Read the model definition and answer for the solid it produces. Units are mm, in the model's axes. Face numbers are marked on the shaded views. A direction names the side the tool comes from. Coordinates: 2 decimals unless noted, no trailing zeros. Order: outer loops, then holes, each group sorted by start corner. A loop starts at its lowest first (then second) coordinate and runs counter-clockwise, first axis right, second up. Notation, with made-up numbers: M 49.5,44.25 L 91.5,44.25 A12 cw 91.5,55.25 Z; hole C 18.5,4 d6. An arc over 180 degrees is marked long. Put each result on its own line as item: value.
from build123d import *

# Parameters (mm, degrees)
F0_W      = 76.2
F0_H      = 76.2
F1_DEPTH  = 25.4
F1_FACE_W = 76.2
F1_FACE_H = 76.2
F2_DEPTH  = 50.8
F3_R      = 25.4
F4_DEPTH  = 25.4
F5_R      = 25.4
F6_DEPTH  = 25.4
F7_W      = 38.1
F7_H      = 38.1
F8_DEPTH  = 101.6


with BuildPart() as f1:
    # F0 (on Front) → F1 (new body)
    with BuildSketch(Plane.XZ):
        with Locations((-36.805706, 34.59075)):
            Rectangle(F0_W, F0_H)
    extrude(amount=F1_DEPTH)

    # F1_face (on face) → F2 (join)
    with BuildSketch(Plane(origin=(-36.805706, -25.4, 34.59075), x_dir=(1, 0, 0), z_dir=(0, -1, 0))):
        Rectangle(F1_FACE_W, F1_FACE_H)
    extrude(amount=F2_DEPTH)

    # F3 (on face) → F4 (join)
    with BuildSketch(Plane.XZ.offset(76.2)):
        with Locations((-36.805706, 34.59075)):
            Circle(F3_R)
    extrude(amount=F4_DEPTH)

    # F5 (on face) → F6 (join)
    with BuildSketch(Plane.YZ.offset(1.294294)):
        with Locations((-38.1, 34.59075)):
            Circle(F5_R)
    extrude(amount=F6_DEPTH)

    # F7 (on face) → F8 (join)
    with BuildSketch(Plane.XY.offset(72.69075)):
        with Locations((-36.805706, -38.1)):
            Rectangle(F7_W, F7_H)
    extrude(amount=F8_DEPTH)


solid = f1.part
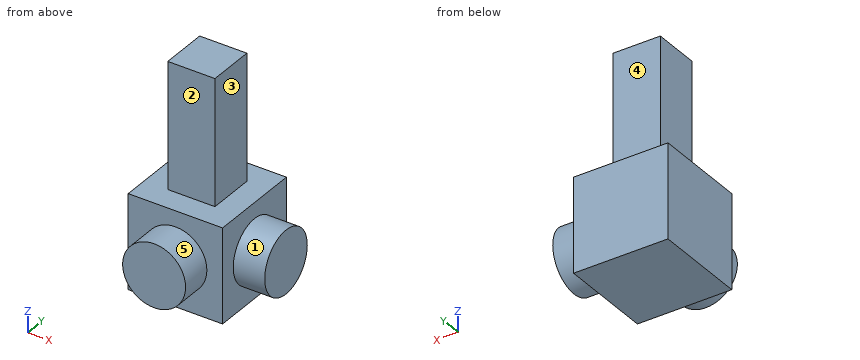
Q1. Find section A-A on y = -38.1. Write down the section's boundary in (x, z), plus the area to 3 significant figures.
Answers below:
outline: M -74.91,-3.51 L 1.29,-3.51 L 1.29,9.19 L 26.69,9.19 L 26.69,59.99 L 1.29,59.99 L 1.29,72.69 L -17.76,72.69 L -17.76,174.29 L -55.86,174.29 L -55.86,72.69 L -74.91,72.69 Z
area: 11,000 mm^2
Q2. Find section C-C on z = 39.5. Write down the section's boundary in (x, y).
Answers below:
outline: M -74.91,-76.2 L -61.73,-76.2 L -61.73,-101.6 L -11.88,-101.6 L -11.88,-76.2 L 1.29,-76.2 L 1.29,-63.02 L 26.69,-63.02 L 26.69,-13.18 L 1.29,-13.18 L 1.29,0 L -74.91,0 Z
Q3. A tool of negligible diameter and unlimited length cuts with its end or side. For the marked faces 1, 2, 3, 4 and 5, from which of +Z, -Z, +X, -X, +Y, -Y can it reach the whole face along a straight path? Write none if from no direction.
Answers below:
face 1: +X
face 2: +Z, +X, -X, -Y
face 3: +Z, +X, +Y, -Y
face 4: +Z, +X, -X, +Y
face 5: -Y
Q4. Consider line 1 along X through (y, z) = (-25.5, 139.5); line 2 along Z through (x, y) = (-28, -6.5); line 3 along Y through (x, z) = (-18, 65). Determine where each line is inside the solid, lowest interval first.
Answers below:
line 1: x = -55.86 to -17.76
line 2: z = -3.51 to 72.69
line 3: y = -76.2 to 0
Q5. Find section B-B on x = -15. Write down the section's boundary in (y, z).
Answers below:
outline: M -101.6,21.56 L -76.2,21.56 L -76.2,-3.51 L 0,-3.51 L 0,72.69 L -76.2,72.69 L -76.2,47.62 L -101.6,47.62 Z
Q6. Given pin 1 (10 mm diameter, centred on y = -34.5, z = 81.5, fed in from -X); pin 2 (6 mm diameter, centred on x = -15.5, z = 122.5, fed in from +Y); pin 3 (19 mm diameter, centred on y = -29.5, z = 146.5, fed in from +X); pin 4 (4 mm diameter, centred on x = -35.5, z = 31, fed in from +Y), each flat-ended and moving along its own axis, determine where each tip first touches the part or whether it passes through.
Answers below:
pin 1: stops at x = -55.86
pin 2: stops at y = -19.05
pin 3: stops at x = -17.76
pin 4: stops at y = 0
Q7. Find section D-D on z = 76. Write down the section's boundary in (x, y), plus the area to 3 significant figures.
Answers below:
outline: M -55.86,-57.15 L -17.76,-57.15 L -17.76,-19.05 L -55.86,-19.05 Z
area: 1,450 mm^2
